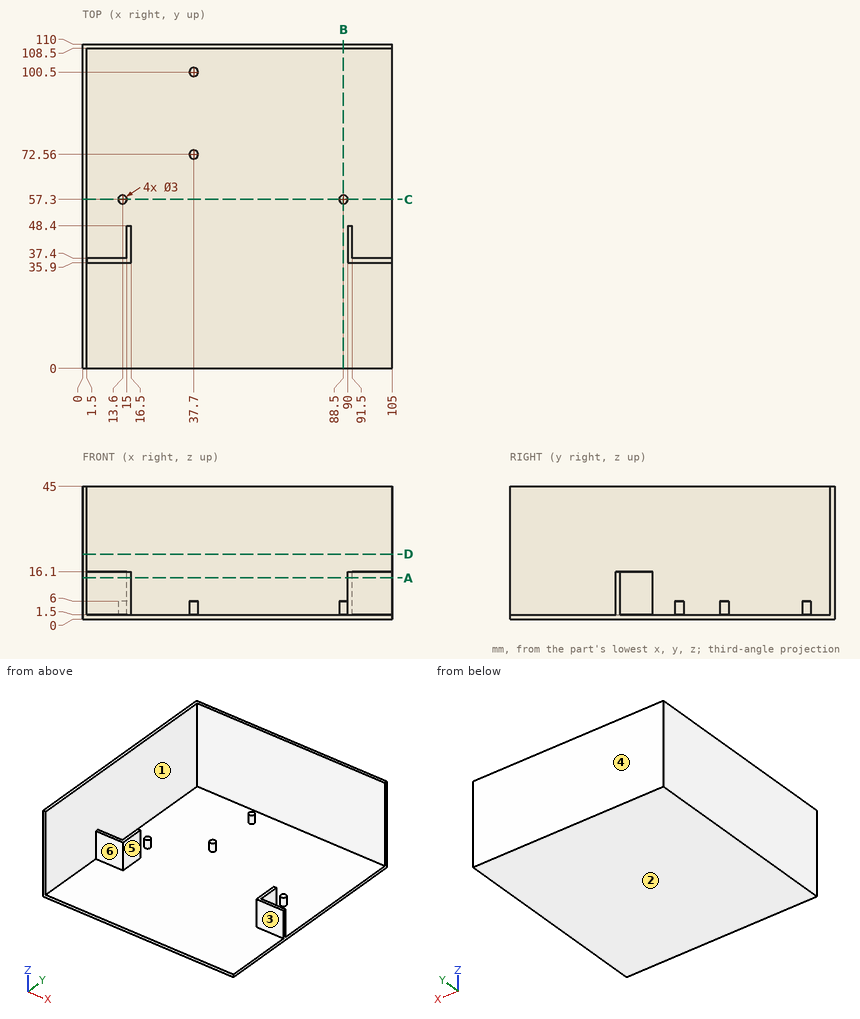
Can you work these out from the drawing? Everything is in mm from the part's minimum corner. A direction names the side the tool comes from. Coordinates: 2 decimals unless noted, no trailing zeros. Loops run counter-clockwise (first coordinate to the right, second up) from the corner with the lowest first, then second, coordinate; pieces in that order, holes last. Notation, with made-up numbers: (-26, 42.5) - (24, 42.5) arc R26 ccw to (24, 67.5) - close; hole circle Ø11 at (5.25, 28). An arc over 180 degrees is marked (long way). Put each result on its own line as item: value. Start each with the question number.
Item 1: Suppose I cut it at D-D (z = 22). Please give me the cut outline in (x, y).
Item 2: For pin 1 (3.5 mm diameter, centred on x = 37.5, y = 73, fed in from +Z); pin 2 (13 mm diameter, centred on y = 59, z = 25, fed in from +X); pin 3 (8 mm diameter, centred on x = 56.5, y = 45.5, fed in from +Z), each with a flat end and sliding along its axis, tell me the tip position at first contact or that it passes through.
Item 3: Suppose I cut it at B-B (x = 88.5). Please give me the cut outline in (y, z), and give its area (3 significant figures).
Item 4: Suppose I cut it at C-C (y = 57.3). Please give me the cut outline in (x, z).
Item 5: If we mould it in two halves opening along Y, with no side actions, what happens to the marked faces 1, 2 and 3? For each: +Y half, -Y half, draft (parallel to the pull), parting line (faces both ways), or undercut.
Item 6: Suppose I cut it at A-A (z = 14). Please give me the cut outline in (x, y), and give its area (3 significant figures).
Item 7: Which directions (+Z, -Z, +X, -X, +Y, -Y) give clear straight access to the entire face, cutting with the end or side of a thin tool? Please do the marked faces 4, 5 and 6.
Item 8: If I drill on line 1 along Y through (x, z) = (6, 13); line 2 along Z through (x, y) = (84, 25), over which ranges is the centre line in solid material (lowest first)?
Here are the results:
1. outline: (0, 0) - (1.5, 0) - (1.5, 108.5) - (105, 108.5) - (105, 110) - (0, 110) - close
2. pin 1: z = 6
2. pin 2: x = 1.5
2. pin 3: z = 1.5
3. outline: (0, 0) - (110, 0) - (110, 45) - (108.5, 45) - (108.5, 1.5) - (58.8, 1.5) - (58.8, 6) - (55.8, 6) - (55.8, 1.5) - (0, 1.5) - close
3. area: 244 mm²
4. outline: (0, 0) - (105, 0) - (105, 1.5) - (90, 1.5) - (90, 6) - (87, 6) - (87, 1.5) - (15.1, 1.5) - (15.1, 6) - (12.1, 6) - (12.1, 1.5) - (1.5, 1.5) - (1.5, 45) - (0, 45) - close
5. face 1: undercut
5. face 2: draft
5. face 3: -Y half
6. outline: (0, 0) - (1.5, 0) - (1.5, 35.9) - (16.5, 35.9) - (16.5, 48.4) - (15, 48.4) - (15, 37.4) - (1.5, 37.4) - (1.5, 108.5) - (105, 108.5) - (105, 110) - (0, 110) - close; (90, 35.9) - (105, 35.9) - (105, 37.4) - (91.5, 37.4) - (91.5, 48.4) - (90, 48.4) - close
6. area: 398 mm²
7. face 4: +Z, -Z, +X, -X, +Y
7. face 5: +Z, -Y
7. face 6: +Z, +X, -Y
8. line 1: 35.9 to 37.4, 108.5 to 110
8. line 2: 0 to 1.5
